Verification items for this drawing (mm, ordinates from the low corner). A direction names the side the tool comes from. Round coordinates to 2 decimals unless told otherwise and drop trailing zeros. Write each loop counter-clockwise with the first axis right and the second up, starting at its lowest first coordinate (ties: lowest second). Pieces come first, ordered by that corner, then holes. Notation, with made-up numbers: (6.5, 83.5) -> (19.5, 83.5) arc R22 cw to (19.5, 122.5) -> close; hole circle Ø3 at (-25.75, 73.25). An arc over 180 degrees is marked (long way). One line per item, written item: value.
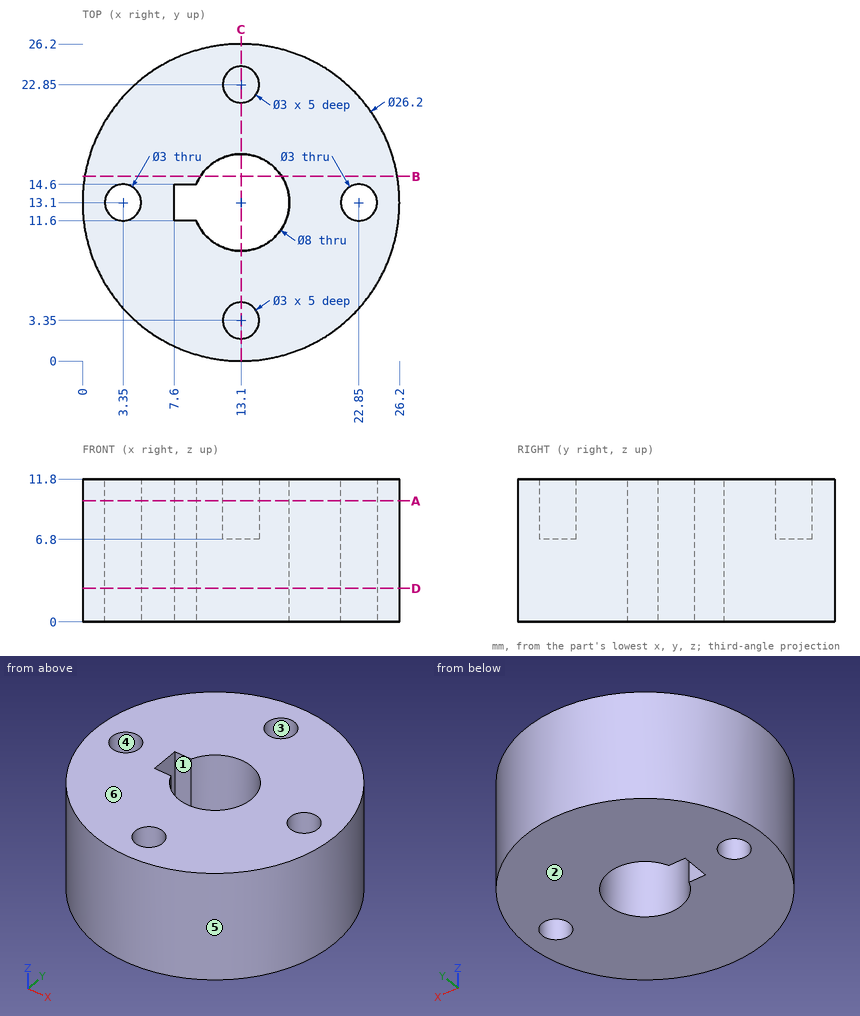
Item 1: Sectioned sample at A-A (z = 10). Enter the section's corners in (x, y).
Result set:
outline: circle Ø26.2 at (13.1, 13.1); hole circle Ø3 at (3.35, 13.1); hole (7.6, 11.6) -> (9.39, 11.6) arc R4 ccw (long way) to (9.39, 14.6) -> (7.6, 14.6) -> close; hole circle Ø3 at (13.1, 3.35); hole circle Ø3 at (13.1, 22.85); hole circle Ø3 at (22.85, 13.1)
Item 2: Material ranges on line 1 along X through (y, z) = (13.5, 7.75); line 2 along X through (y, z) = (12.5, 6.75); line 3 along X through (y, z) = (11.25, 6), recorded low to high.
Result set:
line 1: 0.01 to 1.9, 4.8 to 7.6, 17.08 to 21.4, 24.3 to 26.19
line 2: 0.01 to 1.98, 4.72 to 7.6, 17.05 to 21.48, 24.22 to 26.19
line 3: 0.13 to 9.55, 16.65 to 26.07
Item 3: Sectioned sample at C-C (x = 13.1). Enter the section's corners in (y, z), then the cut area to 3 significant figures.
Result set:
outline: (0, 0) -> (9.1, 0) -> (9.1, 11.8) -> (4.85, 11.8) -> (4.85, 6.8) -> (1.85, 6.8) -> (1.85, 11.8) -> (0, 11.8) -> close; (17.1, 0) -> (26.2, 0) -> (26.2, 11.8) -> (24.35, 11.8) -> (24.35, 6.8) -> (21.35, 6.8) -> (21.35, 11.8) -> (17.1, 11.8) -> close
area: 185 mm^2
Item 4: Sectioned sample at B-B (y = 15.25). Enter the section's corners in (x, z).
Result set:
outline: (0.18, 0) -> (9.73, 0) -> (9.73, 11.8) -> (0.18, 11.8) -> close; (16.47, 0) -> (26.02, 0) -> (26.02, 11.8) -> (16.47, 11.8) -> close
Item 5: Release check for a two-part mould opening along Y. For the marked faces 4, 5 and 6 record: pulls with the +Y half, pulls with the -Y half, needs draft (parallel to the pull), parting line crosses it, or undercut.
Result set:
face 4: undercut
face 5: parting line crosses it
face 6: needs draft
Item 6: Sectioned sample at D-D (z = 2.75). Enter the section's corners in (x, y).
Result set:
outline: circle Ø26.2 at (13.1, 13.1); hole circle Ø3 at (3.35, 13.1); hole (7.6, 11.6) -> (9.39, 11.6) arc R4 ccw (long way) to (9.39, 14.6) -> (7.6, 14.6) -> close; hole circle Ø3 at (22.85, 13.1)
Item 7: Tool access check on the marked faces 1, 2 and 3. Record the directions out of +Z, -Z, +X, -X, +Y, -Y that give a thin tool (end or side, any length) a straight path to the whole face; none if there is none.
Result set:
face 1: +Z, -Z
face 2: -Z, +X, -X, +Y, -Y
face 3: +Z
Item 8: Depth check by flat-ended pin: pin 1 (0.5 mm diameter, centred on x = 8.5, z = 7, fed in from -Y); pin 2 (0.9 mm diameter, centred on x = 13, y = 23.5, fed in from +Z); pin 3 (5 mm diameter, centred on y = 7.5, z = 8.5, fed in from +X). Enter the tip coordinate at first touch or a pass-through.
Result set:
pin 1: y = 0.74
pin 2: z = 6.8
pin 3: x = 25.83
